from build123d import *

# Parameters (mm, degrees)
SKETCH1_R           = 15.875
BOSS_EXTRUDE1_DEPTH = 25.4
SKETCH4_R           = 44.45
BOSS_EXTRUDE2_DEPTH = 7.62
SKETCH6_R           = 2.5527
CUT_EXTRUDE4_DEPTH  = 26.4
CIRPATTERN2_COUNT   = 4
CUT_EXTRUDE5_START  = -11.49604
SKETCH2_R           = 12.7
CUT_EXTRUDE5_DEPTH  = 11.49604
CHAMFER1_SIZE       = 2.38
SKETCH3_R           = 1.7272
CUT_EXTRUDE6_DEPTH  = 26.4


with BuildPart() as part:
    # Sketch1 → Boss-Extrude1 (new body)
    with BuildSketch(Plane(origin=(0, 0, 0), x_dir=(1, 0, 0), z_dir=(0, 1, 0))):
        Circle(SKETCH1_R)
    extrude(amount=BOSS_EXTRUDE1_DEPTH)

    # Sketch4 → Boss-Extrude2 (add)
    with BuildSketch(Plane(origin=(0, 25.4, 0), x_dir=(1, 0, 0), z_dir=(0, 1, 0))):
        Circle(SKETCH4_R)
    extrude(amount=-BOSS_EXTRUDE2_DEPTH)

    # Sketch6 → Cut-Extrude4 (cut, through all)
    with BuildSketch(Plane(origin=(0, 25.4, 0), x_dir=(1, 0, 0), z_dir=(0, 1, 0))):
        with Locations((0, 36.195)):
            Circle(SKETCH6_R)
    cut_extrude4 = extrude(amount=-CUT_EXTRUDE4_DEPTH, mode=Mode.SUBTRACT)

    # CirPattern2: Cut-Extrude4 ×4 about axis
    cirpattern2_axis = Axis((0, 0, 0), (0, 1, 0))
    for i in range(1, CIRPATTERN2_COUNT):
        add(cut_extrude4.rotate(cirpattern2_axis, i * 360 / CIRPATTERN2_COUNT), mode=Mode.SUBTRACT)

    # Sketch2 → Cut-Extrude5 (cut)
    with BuildSketch(Plane(origin=(0, 25.4, 0), x_dir=(1, 0, 0), z_dir=(0, 1, 0)).offset(CUT_EXTRUDE5_START)):
        Circle(SKETCH2_R)
    extrude(amount=CUT_EXTRUDE5_DEPTH, mode=Mode.SUBTRACT)

    # Chamfer1
    chamfer1_edges = [part.edges().sort_by_distance(p)[0] for p in [
        (-15.875, 17.78, 0),
    ]]
    chamfer(chamfer1_edges, length=CHAMFER1_SIZE)

    # Sketch3 → Cut-Extrude6 (cut, through all)
    with BuildSketch(Plane.XZ):
        with Locations((6.735192091, -6.735192091)):
            Circle(SKETCH3_R)
        with Locations((-6.735192091, -6.735192091)):
            Circle(SKETCH3_R)
        with Locations((-6.735192091, 6.735192091)):
            Circle(SKETCH3_R)
        with Locations((6.735192091, 6.735192091)):
            Circle(SKETCH3_R)
    extrude(amount=-CUT_EXTRUDE6_DEPTH, mode=Mode.SUBTRACT)


solid = part.part
Verification items for the finished model (mm, model axes). A direction names the side the tool comes from. Give positions to 0.01 mm unless a question says otherwise; leave off trailing zeros. Write each loop counter-clockwise with the first axis right and the second up, starting at its lowest first coordinate (ties: lowest second). Pieces come first, ordered by that corner, then holes. Notation, with made-up numbers: (69, -30.5) - (82, -30.5) arc R6 ccw to (82, -20.5) - close; hole circle Ø2 at (9.25, -25.75). An arc over 180 degrees is marked (long way). Answer as CSV lines item,"result". Start each with the question number.
1. Depth check by flat-ended pin: pin 1 (6 mm diameter, centred on x = -36.195, z = 0, fed in from -Y); pin 2 (4.5 mm diameter, centred on x = 6.74, z = 6.74, fed in from -Y); pin 3 (7.5 mm diameter, centred on x = -1.5, z = 0, fed in from +Y); pin 4 (10 mm diameter, centred on x = -19.5, z = 11, fed in from -Y). Enter the tip coordinate at first touch or a pass-through.
2. Thickness scan on line 1 (Y direction, x = -16.5, z = 13); line 2 (Z direction, x = 1, y = 23.25); line 3 (Z direction, x = 8, y = 10). Record the ranges inside material, lowest first.
3. Sectioned sample at D-D (y = 21). Record the boundary of the cut face in (x, z) (3 decimals), then the cut area to 3 significant figures.
4. Sectioned sample at C-C (x = 37.5). Record the boundary of the cut face in (y, z).
5. Sectioned sample at A-A (x = 0). Record the boundary of the cut face in (y, z) (3 decimals), then the cut area to 3 significant figures.
6. Set-up check for faces 1 (the face through (-1, 17.78, 19)), 2 (the face through (-8.01, 6.85, 7.9)), 3 (the face through (-2.75, 19.57, 12.4)): record each of +Z, -Z, +X, -X, +Y, -Y from which the full face is reachable in a straight line by a thin tool's end or side.
7. Sectioned sample at B-B (z = 0). Record the boundary of the cut face in (x, y) (3 decimals), then the cut area to 3 significant figures.
Derived:
1,pin 1,"y = 17.78"
1,pin 2,"y = 0"
1,pin 3,"y = 13.9"
1,pin 4,"y = 16.91"
2,line 1,"17.78 to 25.4"
2,line 2,"-44.44 to -38.54, -33.85 to -12.66, 12.66 to 33.85, 38.54 to 44.44"
2,line 3,"-13.71 to -7.91, -5.56 to 5.56, 7.91 to 13.71"
3,outline,"circle Ø88.9 at (0, 0); hole circle Ø5.105 at (-36.195, 0); hole circle Ø25.4 at (0, 0); hole circle Ø5.105 at (0, -36.195); hole circle Ø5.105 at (0, 36.195); hole circle Ø5.105 at (36.195, 0)"
3,area,"5,620 mm²"
4,outline,"(17.78, -23.87) - (25.4, -23.87) - (25.4, -2.19) - (17.78, -2.19) - close; (17.78, 2.19) - (25.4, 2.19) - (25.4, 23.87) - (17.78, 23.87) - close"
5,outline,"(0, -15.875) - (15.4, -15.875) - (17.78, -18.255) - (17.78, -33.642) - (25.4, -33.642) - (25.4, -12.7) - (13.904, -12.7) - (13.904, 12.7) - (25.4, 12.7) - (25.4, 33.642) - (17.78, 33.642) - (17.78, 18.255) - (15.4, 15.875) - (0, 15.875) - close; (17.78, -44.45) - (25.4, -44.45) - (25.4, -38.748) - (17.78, -38.748) - close; (17.78, 38.748) - (25.4, 38.748) - (25.4, 44.45) - (17.78, 44.45) - close"
5,area,"878 mm²"
6,face 1,"-Y"
6,face 2,"+Y, -Y"
6,face 3,"+Y"
7,outline,"(-44.45, 17.78) - (-38.748, 17.78) - (-38.748, 25.4) - (-44.45, 25.4) - close; (-33.642, 17.78) - (-18.255, 17.78) - (-15.875, 15.4) - (-15.875, 0) - (15.875, 0) - (15.875, 15.4) - (18.255, 17.78) - (33.642, 17.78) - (33.642, 25.4) - (12.7, 25.4) - (12.7, 13.904) - (-12.7, 13.904) - (-12.7, 25.4) - (-33.642, 25.4) - close; (38.748, 17.78) - (44.45, 17.78) - (44.45, 25.4) - (38.748, 25.4) - close"
7,area,"878 mm²"
